```python
from build123d import *

# Parameters (mm, degrees)
SKETCH1_W                = 101
SKETCH1_H                = 95.2
SKETCH1_R                = 1.1
SKETCH1_W_2              = 22.3
SKETCH1_H_2              = 10.6
BOSS_EXTRUDE1_DEPTH      = 3
BOSS_EXTRUDE3_DEPTH      = 30
BOSS_EXTRUDE3_DEPTH_BACK = 30
SKETCH5_R                = 2.5
CUT_EXTRUDE1_START       = -40.5
CUT_EXTRUDE1_DEPTH       = 21
SKETCH9_W                = 22.3
SKETCH9_H                = 10.6
CUT_EXTRUDE4_DEPTH       = 10
SKETCH10_W               = 95
SKETCH10_H               = 89.2
BOSS_EXTRUDE4_DEPTH      = 1
CUT_EXTRUDE5_START       = -1.2
SKETCH11_R               = 1.1
SKETCH11_W               = 22.3
SKETCH11_H               = 10.6
CUT_EXTRUDE5_DEPTH       = 1.2


with BuildPart() as part:
    # Sketch1 → Boss-Extrude1 (new body)
    with BuildSketch(Plane.XY):
        Rectangle(SKETCH1_W, SKETCH1_H)
        with Locations((44, 41.1)):
            Circle(SKETCH1_R, mode=Mode.SUBTRACT)
        with Locations((44, -23.9)):
            Circle(SKETCH1_R, mode=Mode.SUBTRACT)
        with Locations((-44, 41.1)):
            Circle(SKETCH1_R, mode=Mode.SUBTRACT)
        with Locations((-44, -23.9)):
            Circle(SKETCH1_R, mode=Mode.SUBTRACT)
        with Locations((-15.65, 32.7)):
            Rectangle(SKETCH1_W_2, SKETCH1_H_2, mode=Mode.SUBTRACT)
        with Locations((15.35, 32.7)):
            Rectangle(SKETCH1_W_2, SKETCH1_H_2, mode=Mode.SUBTRACT)
    extrude(amount=BOSS_EXTRUDE1_DEPTH)

    # Sketch5 → Boss-Extrude3 (add, two sides: drawn at the far end of the back side and taken through both)
    with BuildSketch(Plane(origin=(0, 0, 0), x_dir=(0, -1, 0), z_dir=(-1, 0, 0)).offset(-BOSS_EXTRUDE3_DEPTH_BACK)):
        with BuildLine():
            Line((46.1, 9), (46.1, 3))
            Line((46.1, 3), (25.614718626, 3))
            Line((25.614718626, 3), (-46.1, 3))
            Line((-46.1, 3), (-42.564466094, 6.535533906))
            ThreePointArc((-42.564466094, 6.535533906), (-40.94234935, 7.619397663), (-39.028932188, 8))
            Line((-39.028932188, 8), (28.543650814, 8))
            ThreePointArc((28.543650814, 8), (30.457067976, 8.380602337), (32.07918472, 9.464466094))
            Line((32.07918472, 9.464466094), (35.857359313, 13.242640687))
            ThreePointArc((35.857359313, 13.242640687), (42.396100594, 14.543277195), (46.1, 9))
        make_face()
        with Locations((40.1, 9)):
            Circle(SKETCH5_R, mode=Mode.SUBTRACT)
    extrude(amount=BOSS_EXTRUDE3_DEPTH + BOSS_EXTRUDE3_DEPTH_BACK)

    # Sketch7 → Cut-Extrude1 (cut)
    with BuildSketch(Plane.ZY.offset(30).offset(CUT_EXTRUDE1_START)):
        with BuildLine():
            Line((3, 46.1), (3, -46.1))
            Line((3, -46.1), (9, -46.1))
            ThreePointArc((9, -46.1), (14.543277195, -42.396100594), (13.242640687, -35.857359313))
            Line((13.242640687, -35.857359313), (9.464466094, -32.07918472))
            ThreePointArc((9.464466094, -32.07918472), (8.380602337, -30.457067976), (8, -28.543650814))
            Line((8, -28.543650814), (8, 39.028932188))
            ThreePointArc((8, 39.028932188), (7.619397663, 40.94234935), (6.535533906, 42.564466094))
            Line((6.535533906, 42.564466094), (3, 46.1))
        make_face()
    extrude(amount=CUT_EXTRUDE1_DEPTH, mode=Mode.SUBTRACT)

    # Sketch9 → Cut-Extrude4 (cut)
    with BuildSketch(Plane.XY.offset(3)):
        with Locations((15.35, 32.7)):
            Rectangle(SKETCH9_W, SKETCH9_H)
        with Locations((-15.65, 32.7)):
            Rectangle(SKETCH9_W, SKETCH9_H)
    extrude(amount=CUT_EXTRUDE4_DEPTH, mode=Mode.SUBTRACT)

    # Sketch10 → Boss-Extrude4 (add)
    with BuildSketch(Plane(origin=(0, 0, 0), x_dir=(-1, 0, 0), z_dir=(0, 0, -1))):
        Rectangle(SKETCH10_W, SKETCH10_H)
    extrude(amount=BOSS_EXTRUDE4_DEPTH)

    # Sketch11 → Cut-Extrude5 (cut)
    with BuildSketch(Plane.XY.offset(CUT_EXTRUDE5_START)):
        with Locations(Location((-44, 41.1, 0), (0, 0, 180))):
            Circle(SKETCH11_R)
        with Locations(Location((-44, -23.9, 0), (0, 0, 180))):
            Circle(SKETCH11_R)
        with Locations(Location((44, -23.9, 0), (0, 0, 180))):
            Circle(SKETCH11_R)
        with Locations(Location((44, 41.1, 0), (0, 0, 180))):
            Circle(SKETCH11_R)
        with Locations((15.35, 32.7)):
            Rectangle(SKETCH11_W, SKETCH11_H)
        with Locations((-15.65, 32.7)):
            Rectangle(SKETCH11_W, SKETCH11_H)
    extrude(amount=CUT_EXTRUDE5_DEPTH, mode=Mode.SUBTRACT)


solid = part.part
```
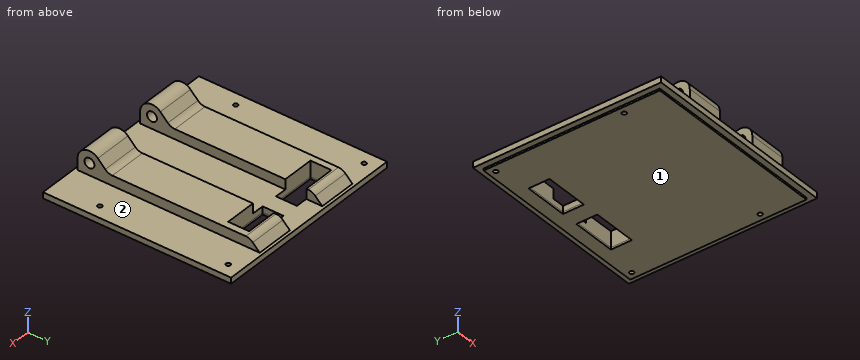
The listing builds one solid part. Answer for the finished solid, in the listing's coordinates (mm). Face numbers are marked on the shaded views. Coordinates: 2 decimals unless noted, no trailing zeros. Loops run counter-clockwise (first coordinate to the right, second up) from the corner with the lowest first, then second, coordinate; pieces in that order, holes last. Notation, with made-up numbers: M 45.25,10.5 L 58.25,10.5 A27 cw 58.25,34.5 Z; hole C 9,41 d6. An arc over 180 degrees is marked long. Answer as a JSON object with one key per item and string values. Group by question number.
Item 1: Determine the mould class of the marked faces 1 and 2 for opening direction X: +X half, -X half, draft (parallel to the pull), parting line (faces both ways), or undercut.
Item 2: Each of these flat-tipped pins is pushed along its axis until it touches: P1, Ø3, axis at x = -44, y = -23.9, coming from the +Z side; P2, Ø8, axis at y = -40.1, z = 9, coming from the -X side; P3, Ø0.8, axis at x = 19, z = -0.5, coming from the -Y side; P4, Ø1.3, axis at x = -44, y = -23.9, coming from the -Z side. Where does it stop, or does it pass through?
Item 3: Section D-D (z = 1.25) is taken. Write down the section's boundary in (x, y).
Item 4: Consider L1, parallel to X at y = -23.9, z = -0.2; L2, parallel to Y at x = 44, z = -0.75; L3, parallel to Y at x = -44, z = 1.2. Determine where each line is inside the solid, lowest interval first.
Item 5: Section A-A (x = 18) is taken. Write down the section's boundary in (y, z).
Item 6: Section C-C (x = 6) is taken. Write down the section's boundary in (y, z), and give its area (3 significant figures).
Item 7: Section B-B (y = -40.1) is taken. Write down the section's boundary in (x, z), and give its area (3 significant figures).
Solved:
{
 "1": {"face 1": "draft", "face 2": "undercut"},
 "2": {"P1": "stops at z = 3", "P2": "stops at x = -30", "P3": "stops at y = -44.6", "P4": "passes through"},
 "3": {"outline": "M -50.5,-47.6 L 50.5,-47.6 L 50.5,47.6 L -50.5,47.6 Z; hole C -44,-23.9 d2.2; hole C -44,41.1 d2.2; hole M -26.8,27.4 L -4.5,27.4 L -4.5,38 L -26.8,38 Z; hole M 4.2,27.4 L 26.5,27.4 L 26.5,38 L 4.2,38 Z; hole C 44,-23.9 d2.2; hole C 44,41.1 d2.2"},
 "4": {"L1": "x = -47.5 to -45.1, -42.9 to 42.9, 45.1 to 47.5", "L2": "y = -44.6 to -25, -22.8 to 40, 42.2 to 44.6", "L3": "y = -47.6 to -25, -22.8 to 40, 42.2 to 47.6"},
 "5": {"outline": "M -47.6,0 L -44.6,0 L -44.6,-1 L 27.4,-1 L 27.4,8 L -28.54,8 A5 cw -32.08,9.46 L -35.86,13.24 A6 ccw -46.1,9 L -46.1,3 L -47.6,3 Z; M 38,-1 L 44.6,-1 L 44.6,0 L 47.6,0 L 47.6,3 L 46.1,3 L 42.56,6.54 A5 ccw 39.03,8 L 38,8 Z; hole C -40.1,9 d5"},
 "6": {"outline": "M -47.6,0 L -44.6,0 L -44.6,-1 L 27.4,-1 L 27.4,3 L -47.6,3 Z; M 38,-1 L 44.6,-1 L 44.6,0 L 47.6,0 L 47.6,3 L 38,3 Z", "area": "332 mm2"},
 "7": {"outline": "M -50.5,0 L -47.5,0 L -47.5,-1 L 47.5,-1 L 47.5,0 L 50.5,0 L 50.5,3 L 30,3 L 30,6.5 L 10.5,6.5 L 10.5,3 L -10.5,3 L -10.5,6.5 L -30,6.5 L -30,3 L -50.5,3 Z; M -30,11.5 L -10.5,11.5 L -10.5,15 L -30,15 Z; M 10.5,11.5 L 30,11.5 L 30,15 L 10.5,15 Z", "area": "671 mm2"}
}
